Can you work these out from the model? Positions are in its coordinate system, mm. A direction names the side the tool comes from. Round coordinates to 2 decimals unless told otherwise and drop trailing zeros. Order: outer loops, then holes, each group sorted by start corner. A loop starts at its lowest first (then second) coordinate and runs counter-clockwise, first axis right, second up. Notation, with made-up numbers: (11.25, -15.75) -> (67.25, -15.75) arc R21 ccw to (67.25, -11.75) -> close; hole circle Ø8 at (-20, 64). An arc over 180 degrees is marked (long way). Use a Markdown table: item, result. Add a question column.
Q1. We'd pull the mould along X, two halves only. Please class faces 3 (the face through (-45, 36, 9)), 4 (the face through (-75, 1, 9)), 5 (the face through (-60, 50, 7)): +X half, -X half, draft (parallel to the pull), parting line (faces both ways), or undercut.
Q2. I'm going to push a flat-ended pin straight in: pin 1 Ø1 at (x, z) = (-23, 6.5) entering from +Y. Where does the tip first touch, or does it pass through?
Q3. If we section it at D-D on x = 13: List the corners of the cut face in (y, z) for me.
Q4. I need wall thicknesses on line 1 along Z through (x, y) = (64.75, 40.5); line 2 along X through (y, z) = (45.5, 10.5); line 3 along Y through (x, z) = (11, 4.5). Which ranges of each line are inside material? Lowest first, please. Write a range as [from, to].
Q5. For faces 1 (the face through (45, 37, 7)), 2 (the face through (-1, -50, 9)), which set-ups out of +Z, -Z, +X, -X, +Y, -Y let a thin tool reach every point of the face, with its end or its side?
Q6. If we section it at B-B on y = 40.5: List the corners of the cut face in (x, z) for me, plus the area to 3 significant figures.
Q7. If we section it at C-C on z = 17.5: List the corners of the cut face in (x, y) for me.
Q8. If we section it at A-A on z = 9.5: List the corners of the cut face in (x, y) for me, plus the area to 3 significant figures.
```python
from build123d import *

# Parameters (mm, degrees)
F1_DEPTH = 19
F2_R     = 4
F3_DEPTH = 150.001
F4_R     = 5


with BuildPart() as f1:
    # F0 (on Top) → F1 (new body)
    with BuildSketch(Plane.XY):
        Polygon((-75, -50), (75, -50), (75, 50), (45, 50), (45, 28), (-45, 28), (-45, 50), (-75, 50), align=None)
    extrude(amount=F1_DEPTH)

    # F2 (on face) → F3 (cut, through all)
    with BuildSketch(Plane.YZ.offset(75)):
        with Locations((40.5, 9.5)):
            Circle(F2_R)
    extrude(amount=-F3_DEPTH, mode=Mode.SUBTRACT)

    # F4
    f4_edges = [f1.edges().sort_by_distance(p)[0] for p in [
        (-60, 50, 19),
        (60, 50, 19),
    ]]
    fillet(f4_edges, radius=F4_R)


solid = f1.part
```
Answer below:
| question | item | result |
|---|---|---|
| 1 | face 3 | undercut |
| 1 | face 4 | -X half |
| 1 | face 5 | draft |
| 2 | pin 1 | y = 28 |
| 3 | outline | (-50, 0) -> (28, 0) -> (28, 19) -> (-50, 19) -> close |
| 4 | line 1 | [0, 5.5], [13.5, 19] |
| 4 | line 2 | [-75, -45], [45, 75] |
| 4 | line 3 | [-50, 28] |
| 5 | face 1 | +Z, -Z, +Y |
| 5 | face 2 | +Z, -Z, +X, -X, -Y |
| 6 | outline | (-75, 0) -> (-45, 0) -> (-45, 5.5) -> (-75, 5.5) -> close; (-75, 13.5) -> (-45, 13.5) -> (-45, 19) -> (-75, 19) -> close; (45, 0) -> (75, 0) -> (75, 5.5) -> (45, 5.5) -> close; (45, 13.5) -> (75, 13.5) -> (75, 19) -> (45, 19) -> close |
| 6 | area | 660 mm² |
| 7 | outline | (-75, -50) -> (75, -50) -> (75, 48.57) -> (45, 48.57) -> (45, 28) -> (-45, 28) -> (-45, 48.57) -> (-75, 48.57) -> close |
| 8 | outline | (-75, -50) -> (75, -50) -> (75, 36.5) -> (45, 36.5) -> (45, 28) -> (-45, 28) -> (-45, 36.5) -> (-75, 36.5) -> close; (-75, 44.5) -> (-45, 44.5) -> (-45, 50) -> (-75, 50) -> close; (45, 44.5) -> (75, 44.5) -> (75, 50) -> (45, 50) -> close |
| 8 | area | 12,500 mm² |
